The listing builds one solid part. Answer for the finished solid, in the listing's coordinates (mm). A direction names the side the tool comes from. Give positions to 0.01 mm unless a question says otherwise; leave off trailing zeros. Order: outer loops, then holes, each group sorted by start corner. A loop starts at its lowest first (then second) coordinate and runs counter-clockwise, first axis right, second up. Notation, with made-up numbers: (-39, 83.25) - (4, 83.25) arc R15 cw to (4, 109.25) - close; hole circle Ø3 at (-20, 22.5). An arc over 180 degrees is marked (long way). Write each question's results on one line, items separated by ' | '. Start each with the question number.
1. Find the intervals of material crossed by L1, parallel to Y at x = 0.5, z = 6; L2, parallel to Z at x = 13.5, y = -29.5; L3, parallel to X at y = -9, z = 3, in increasing order.
2. Section D-D (z = 17) is taken. Give the vertices of the cut face in (x, y).
3. Section A-A (y = 0) is taken. Give the vertices of the cut face in (x, z), and give its area (3 significant figures).
4. Determine the mould class of faces 1 (the face through (20.5, -22.9, 0.8)), 2 (the face through (28, 6, 1)), 3 (the face through (0, -26, 1.5)) for opening direction X: released by +X, released by -X, zero draft, split by the parting line, or undercut.
5. Section C-C (x = -8) is taken. Give the vertices of the cut face in (y, z).
6. Which of the six approach directions +Z, -Z, +X, -X, +Y, -Y give full straight-line access (tool end or side, diameter ignored) to faces 4 (the face through (26, 0, 2)), 5 (the face through (0, -19, 11)), 6 (the face through (18.9, -26, 1))?
7. Section B-B (x = 20.5) is taken. Give the vertices of the cut face in (y, z).
8. Flat-ended cylindrical pins translate along their axes: pin 1 (10 mm diameter, centred on y = -19.5, z = 6.5, fed in from -X); pin 2 (1.2 mm diameter, centred on y = -25.5, z = 0.5, fed in from +X); pin 3 (1.5 mm diameter, centred on x = 19.5, y = -20.5, fed in from +Z). Find the tip coordinate at first contact, or state that the pin passes through.
from build123d import *

# Parameters (mm, degrees)
ESQUISSE1_W             = 50
ESQUISSE1_H             = 38
BOSS_EXTRU_1_DEPTH      = 20
ESQUISSE2_W             = 50
ESQUISSE2_H             = 1.5
BOSS_EXTRU_2_DEPTH      = 15
CONG_1_R                = 2
ENL_V_MAT_EXTRU_1_DEPTH = 47.078736962
ESQUISSE4_R             = 1.5
BOSS_EXTRU_3_DEPTH      = 2
CONG_2_R                = 4


with BuildPart() as part:
    # Esquisse1 → Boss.-Extru.1 (new body)
    with BuildSketch(Plane.XY):
        Rectangle(ESQUISSE1_W, ESQUISSE1_H)
    extrude(amount=BOSS_EXTRU_1_DEPTH)

    # Esquisse2 → Boss.-Extru.2 (add)
    with BuildSketch(Plane(origin=(0, -19, 0), x_dir=(-1, 0, 0), z_dir=(0, -1, 0))):
        with Locations((0, -0.75)):
            Rectangle(ESQUISSE2_W, ESQUISSE2_H)
    extrude(amount=BOSS_EXTRU_2_DEPTH)

    # Congé1
    cong_1_edges = [part.edges().sort_by_distance(p)[0] for p in [
        (-25, -34, 0.75),
        (25, -34, 0.75),
    ]]
    fillet(cong_1_edges, radius=CONG_1_R)

    # Esquisse3 → Enlèv. mat.-Extru.1 (cut, through all)
    with BuildSketch(Plane.XY.offset(1.5)):
        with BuildLine():
            Line((-22.1, -24.5), (-22.1, -27.5))
            ThreePointArc((-22.1, -27.5), (-20.5, -29.1), (-18.9, -27.5))
            Line((-18.9, -27.5), (-18.9, -24.5))
            ThreePointArc((-18.9, -24.5), (-20.5, -22.9), (-22.1, -24.5))
        make_face()
        with BuildLine():
            Line((18.9, -24.5), (18.9, -27.5))
            ThreePointArc((18.9, -27.5), (20.5, -29.1), (22.1, -27.5))
            Line((22.1, -27.5), (22.1, -24.5))
            ThreePointArc((22.1, -24.5), (20.5, -22.9), (18.9, -24.5))
        make_face()
    extrude(amount=-ENL_V_MAT_EXTRU_1_DEPTH, mode=Mode.SUBTRACT)

    # Esquisse4 → Boss.-Extru.3 (add)
    # profile 1 of 2: a face of its own
    with BuildSketch(Plane(origin=(0, 0, 0), x_dir=(-1, 0, 0), z_dir=(0, 0, -1))):
        Polygon((-25, 9), (-34, 0), (-25, -9), align=None)
        with Locations((-28.5, 0)):
            Circle(ESQUISSE4_R, mode=Mode.SUBTRACT)
    # profile 2 of 2: a face of its own
    with BuildSketch(Plane(origin=(0, 0, 0), x_dir=(-1, 0, 0), z_dir=(0, 0, -1))):
        Polygon((25, -9), (34, 0), (25, 9), align=None)
        with Locations((28.5, 0)):
            Circle(ESQUISSE4_R, mode=Mode.SUBTRACT)
    extrude(amount=-BOSS_EXTRU_3_DEPTH)

    # Congé2
    cong_2_edges = [part.edges().sort_by_distance(p)[0] for p in [
        (34, 0, 1),
        (-34, 0, 1),
    ]]
    fillet(cong_2_edges, radius=CONG_2_R)


solid = part.part
Reported:
1) L1: -19 to 19 | L2: 0 to 1.5 | L3: -25 to 25
2) outline: (-25, -19) - (25, -19) - (25, 19) - (-25, 19) - close
3) outline: (-32.34, 0) - (-30, 0) - (-30, 2) - (-32.34, 2) - close; (-27, 0) - (27, 0) - (27, 2) - (25, 2) - (25, 20) - (-25, 20) - (-25, 2) - (-27, 2) - close; (30, 0) - (32.34, 0) - (32.34, 2) - (30, 2) - close | area: 1,020 mm²
4) face 1: undercut | face 2: released by +X | face 3: zero draft
5) outline: (-34, 0) - (19, 0) - (19, 20) - (-19, 20) - (-19, 1.5) - (-34, 1.5) - close
6) face 4: +Z, +X, +Y, -Y | face 5: +Z, +X, -X, -Y | face 6: +Z, -Z
7) outline: (-34, 0) - (-29.1, 0) - (-29.1, 1.5) - (-34, 1.5) - close; (-22.9, 0) - (19, 0) - (19, 20) - (-19, 20) - (-19, 1.5) - (-22.9, 1.5) - close
8) pin 1: x = -25 | pin 2: x = 25 | pin 3: z = 1.5
